from build123d import *

# Parameters (mm, degrees)
F0_W      = 88.8
F0_H      = 26
F1_DEPTH  = 60
F3_DEPTH  = 45
F4_R      = 2
F5_W      = 88.9
F5_H      = 40
F6_DEPTH  = 10
F8_DEPTH  = 10
F9_R      = 2
F10_W     = 89
F10_H     = 45
F11_DEPTH = 15
F13_DEPTH = 5
F14_R     = 2
F15_R     = 4.6723110677
F15_R_2   = 4
F16_DEPTH = 85.001
F17_W     = 79.5239582658
F17_H     = 118.802215904
F18_DEPTH = 80
F19_R     = 3
F20_DEPTH = 3.2
F20_TAPER = -3
F21_R     = 4.232200224
F22_DEPTH = 25
F22_TAPER = -3


with BuildPart() as f1:
    # F0 (on Top) → F1 (new body)
    with BuildSketch(Plane.XY):
        Rectangle(F0_W, F0_H)
    extrude(amount=F1_DEPTH)

    # F2 (on face) → F3 (cut)
    with BuildSketch(Plane(origin=(0, 0, 0), x_dir=(1, 0, 0), z_dir=(0, 0, -1))):
        Polygon((-17.5, -7.6945363638), (0, -8), (17.5, -7.6945363638), (17.5, 7.6945363638), (0, 8), (-17.5, 7.6945363638), align=None)
    extrude(amount=-F3_DEPTH, mode=Mode.SUBTRACT)

    # F4
    f4_edges = [f1.edges().sort_by_distance(p)[0] for p in [
        (-17.5, 7.694536, 22.5),
        (-17.5, -7.694536, 22.5),
        (17.5, -7.694536, 22.5),
        (17.5, 7.694536, 22.5),
    ]]
    fillet(f4_edges, radius=F4_R)

    # F5 (on face) → F6 (join)
    with BuildSketch(Plane(origin=(0, 0, 0), x_dir=(1, 0, 0), z_dir=(0, 0, -1))):
        Rectangle(F5_W, F5_H)
    extrude(amount=F6_DEPTH)

    # F7 (on face) → F8 (cut)
    with BuildSketch(Plane(origin=(0, 0, -10), x_dir=(1, 0, 0), z_dir=(0, 0, -1))):
        Polygon((-20, -10.1508987014), (0, -10.5), (20, -10.1508987014), (20, 10.1508987014), (0, 10.5), (-20, 10.1508987014), align=None)
    extrude(amount=-F8_DEPTH, mode=Mode.SUBTRACT)

    # F9
    f9_edges = [f1.edges().sort_by_distance(p)[0] for p in [
        (-20, 10.150899, -5),
        (-20, -10.150899, -5),
        (20, 10.150899, -5),
        (20, -10.150899, -5),
    ]]
    fillet(f9_edges, radius=F9_R)

    # F10 (on face) → F11 (join)
    with BuildSketch(Plane(origin=(0, 0, -10), x_dir=(1, 0, 0), z_dir=(0, 0, -1))):
        Rectangle(F10_W, F10_H)
    extrude(amount=F11_DEPTH)

    # F12 (on face) → F13 (cut)
    with BuildSketch(Plane.XY.offset(-10)):
        Polygon((-39.5, -16.5605249353), (0, -17.25), (39.5, -16.5605249353), (39.5, 16.5605249353), (0, 17.25), (-39.5, 16.5605249353), align=None)
    extrude(amount=-F13_DEPTH, mode=Mode.SUBTRACT)

    # F14
    f14_edges = [f1.edges().sort_by_distance(p)[0] for p in [
        (-39.5, 16.560525, -12.5),
        (-39.5, -16.560525, -12.5),
        (39.5, -16.560525, -12.5),
        (39.5, 16.560525, -12.5),
    ]]
    fillet(f14_edges, radius=F14_R)

    # F15 (on face) → F16 (cut, through all)
    with BuildSketch(Plane.XY.offset(60)):
        with Locations((-27.5, 0)):
            Circle(F15_R)
        with Locations((27.5, 0)):
            Circle(F15_R_2)
    extrude(amount=-F16_DEPTH, mode=Mode.SUBTRACT)

    # F17 (on Right) → F18 (cut)
    with BuildSketch(Plane.YZ):
        with Locations((3.9665214717, 9.8679382354)):
            Rectangle(F17_W, F17_H)
    extrude(amount=-F18_DEPTH, mode=Mode.SUBTRACT)

    # F19 (on face) → F20 (cut)
    with BuildSketch(Plane(origin=(0, 0, 0), x_dir=(0, -1, 0), z_dir=(-1, 0, 0))):
        with Locations((0, 53.2094612718)):
            Circle(F19_R)
        with Locations((0, -20.896807313)):
            Circle(F19_R)
    extrude(amount=-F20_DEPTH, taper=F20_TAPER, mode=Mode.SUBTRACT)

    # F21 (on face) → F22 (cut)
    with BuildSketch(Plane(origin=(0, 0, 45), x_dir=(1, 0, 0), z_dir=(0, 0, -1))):
        with Locations((9.2245656997, 0)):
            Circle(F21_R)
    extrude(amount=-F22_DEPTH, taper=F22_TAPER, mode=Mode.SUBTRACT)


solid = f1.part
Source: CAD feature listing. Evaluate the final solid. Frame: model axes, mm. A direction names the side the tool comes from. Coordinates: 2 decimals unless noted, no trailing zeros. Loops run counter-clockwise (first coordinate to the right, second up) from the corner with the lowest first, then second, coordinate; pieces in that order, holes last. Notation, with made-up numbers: M -3,22.25 L 20,22.25 A13 ccw 20,34.25 Z; hole C 79,-26.75 d1. An arc over 180 degrees is marked long. Answer in a Markdown table with one row per item.
Q1. First-contact query: pin 1 (3 mm diameter, centred on x = 26.5, z = -4.5, fed in from -Y); pin 2 (3 mm diameter, centred on y = -3, z = -5, fed in from -X); pin 3 (1.5 mm diameter, centred on y = -6, z = -13, fed in from -X); pin 4 (6.5 mm diameter, centred on x = 27.5, y = 0, fed in from -Z). Flat tips, straight axial feed; report the tip coordinate or a pass-through.
Answers below:
| item | result |
|---|---|
| pin 1 | stops at y = -20 |
| pin 2 | stops at x = 20 |
| pin 3 | stops at x = 39.5 |
| pin 4 | passes through |
Q2. Draft query along Y for faces 5 (the flat face through (4.7, -0.1, 45)), 6 (the flat face through (22, 13, 30)), 7 (the flat face through (22, 0, 60)). Return one class per face: pulls with the +Y half, pulls with the -Y half, needs draft (parallel to the pull), parting line crosses it, or undercut.
Answers below:
| item | result |
|---|---|
| face 5 | undercut |
| face 6 | pulls with the +Y half |
| face 7 | needs draft |
Q3. Section B-B on x = 27.5. Return the cut outline in (y, z).
Answers below:
| item | result |
|---|---|
| outline | M -22.5,-25 L -4,-25 L -4,-15 L -16.77,-15 L -16.77,-10 L -4,-10 L -4,60 L -13,60 L -13,0 L -20,0 L -20,-10 L -22.5,-10 Z; M 4,-25 L 22.5,-25 L 22.5,-10 L 20,-10 L 20,0 L 13,0 L 13,60 L 4,60 L 4,-10 L 16.77,-10 L 16.77,-15 L 4,-15 Z |
Q4. Section D-D on z = -12. Return the cut outline in (x, y), plus the area to 3 significant figures.
Answers below:
| item | result |
|---|---|
| outline | M 0,-22.5 L 44.5,-22.5 L 44.5,22.5 L 0,22.5 L 0,17.25 L 37.53,16.59 A2 cw 39.5,14.6 L 39.5,-14.6 A2 cw 37.53,-16.59 L 0,-17.25 Z |
| area | 669 mm^2 |
Q5. Ray query, probe 1 along Z at (x, y) = (27.5, -7); probe 2 along Z at (x, y) = (34.5, 15); probe 3 along Y at (x, z) = (27.5, 26.5). Return the intervals inside material, ascending. Write a range as from..to.
Answers below:
| item | result |
|---|---|
| probe 1 | z = -25..-15, -10..60 |
| probe 2 | z = -25..-15, -10..0 |
| probe 3 | y = -13..-4, 4..13 |
Q6. Section C-C on x = 34. Return the cut outline in (y, z).
Answers below:
| item | result |
|---|---|
| outline | M -22.5,-25 L 22.5,-25 L 22.5,-10 L 20,-10 L 20,0 L 13,0 L 13,60 L -13,60 L -13,0 L -20,0 L -20,-10 L -22.5,-10 Z; hole M -16.66,-15 L 16.66,-15 L 16.66,-10 L -16.66,-10 Z |
Q7. Set-up query: faces 1 (the flat face through (44.4, 0, 30)), 2 (the flat face through (24, 4, -10)), 3 (the flat face through (0, 10, 18)), 4 (the conical face through (1.62, 0.4, 56.27)). Return all of +Z, -Z, +X, -X, +Y, -Y with unobstructed straight access to the full face (end or side cutting, diameter ignored); none if empty.
Answers below:
| item | result |
|---|---|
| face 1 | +Z, +X, +Y, -Y |
| face 2 | -X |
| face 3 | +Z, -Z, -X, +Y, -Y |
| face 4 | none |
Q8. Section A-A on z = 24. Return the cut outline in (x, y).
Answers below:
| item | result |
|---|---|
| outline | M 0,-13 L 44.4,-13 L 44.4,13 L 0,13 L 0,8 L 15.53,7.73 A2 cw 17.5,5.73 L 17.5,-5.73 A2 cw 15.53,-7.73 L 0,-8 Z; hole C 27.5,0 d8 |
